from build123d import *

# Parameters (mm, degrees)
SKETCH_1_R                           = 20
EXTRUDE_1_DEPTH                      = 5
CUT_EXTRUDE_START                    = -5
SKETCH_4_R                           = 2.75
CUT_EXTRUDE_3_DEPTH                  = 15
SKETCH_7_R                           = 2.3
EXTRUDE_3_DEPTH                      = 4.5
CHAMFER_3_SIZE                       = 0.5
PATTERN_CIRCULAR_1_COUNT             = 4
CHAMFER_3_OF_PATTERN_CIRCULAR_1_SIZE = 0.5
CHAMFER_4_SIZE                       = 0.3
CHAMFER_5_SIZE                       = 1


with BuildPart() as part:
    # 草图1 → 凸台-拉伸1 (new body)
    with BuildSketch(Plane(origin=(0, 0, 0), x_dir=(1, 0, 0), z_dir=(0, 1, 0))):
        with Locations(Location((0, 0, 0), (0, 0, 270))):
            Circle(SKETCH_1_R)
    extrude(amount=EXTRUDE_1_DEPTH)

    # 草图4 → 切除-拉伸3 (cut)
    with BuildSketch(Plane(origin=(0, 5, 0), x_dir=(1, 0, 0), z_dir=(0, 1, 0)).offset(CUT_EXTRUDE_START)):
        with Locations(Location((0, 0, 0), (0, 0, 270))):
            Circle(SKETCH_4_R)
    extrude(amount=CUT_EXTRUDE_3_DEPTH, mode=Mode.SUBTRACT)

    # 草图7 → 凸台-拉伸3 (add)
    with BuildSketch(Plane(origin=(0, 5, 0), x_dir=(1, 0, 0), z_dir=(0, 1, 0))):
        with Locations(Location((6, 0, 0), (0, 0, 270))):
            Circle(SKETCH_7_R)
    extrude_3 = extrude(amount=EXTRUDE_3_DEPTH)

    # 倒角3
    chamfer_3_edges = [part.edges().sort_by_distance(p)[0] for p in [
        (6, 5, -2.3),
        (6, 9.5, -2.3),
    ]]
    chamfer(chamfer_3_edges, length=CHAMFER_3_SIZE)

    # 阵列(圆周)1: 凸台-拉伸3 ×4 about axis
    pattern_circular_1_axis = Axis((0, 0, 0), (0, 1, 0))
    for i in range(1, PATTERN_CIRCULAR_1_COUNT):
        add(extrude_3.rotate(pattern_circular_1_axis, i * 360 / PATTERN_CIRCULAR_1_COUNT))

    # 倒角3 of 阵列(圆周)1
    chamfer_3_of_pattern_circular_1_edges = [part.edges().sort_by_distance(p)[0] for p in [
        (-2.3, 5, -6),
        (-2.3, 9.5, -6),
        (-6, 5, 2.3),
        (-6, 9.5, 2.3),
        (2.3, 5, 6),
        (2.3, 9.5, 6),
    ]]
    chamfer(chamfer_3_of_pattern_circular_1_edges, length=CHAMFER_3_OF_PATTERN_CIRCULAR_1_SIZE)

    # 倒角4
    chamfer_4_edges = [part.edges().sort_by_distance(p)[0] for p in [
        (0, 5, -2.75),
        (0, 0, -2.75),
    ]]
    chamfer(chamfer_4_edges, length=CHAMFER_4_SIZE)

    # 倒角5
    chamfer_5_edges = [part.edges().sort_by_distance(p)[0] for p in [
        (0, 0, -20),
        (0, 5, -20),
    ]]
    chamfer(chamfer_5_edges, length=CHAMFER_5_SIZE)


solid = part.part
Model file for the job. Use its own axes, mm. A direction names the side the tool comes from. Give positions to 0.01 mm unless a question says otherwise; leave off trailing zeros. Loops run counter-clockwise (first coordinate to the right, second up) from the corner with the lowest first, then second, coordinate; pieces in that order, holes last. Notation, with made-up numbers: (19, -18.5) -> (33, -18.5) arc R16 cw to (33, 3.5) -> close; hole circle Ø7 at (-31.5, 40.5). An arc over 180 degrees is marked (long way). Use a Markdown table: item, result. Add a question column.
(1) Slice it at C-C on y = 3.25. List the corners of the cut face in (x, z).
(2) Wall check: line 1 along Z through (x, y) = (0, 6); line 2 along X through (y, z) = (1.7, 0); line 3 along Y through (x, z) = (16.5, 2.5). Give the ranges that are in metal, low to high.
(3) Mould opens along Z. For faces 1 (the flat face through (0, 9.5, -6)), 2 (the cylindrical face through (-19.524, 2.479, -4.336)), 3 (the cylindrical face through (0.499, 7.226, 3.755)) say: +Z half, -Z half, draft (parallel to the pull), parting line (faces both ways), or undercut.
(4) Tool access for faces 4 (the flat face through (-6, 9.5, 0)), 5 (the cylindrical face through (-0.499, 7.226, -3.755)): list every direction of +Z, -Z, +X, -X, +Y, -Y with a clear straight run to the whole face (end or side of a thin tool).
(5) Slice it at B-B on y = 7.75. List the corners of the cut face in (x, z).
(6) Drop flat-ended pins along their axis: pin 1 Ø2 at (x, z) = (12, 7.5) entering from +Y; pin 2 Ø1.5 at (x, y) = (15.5, 5.5) entering from -Z; pin 3 Ø2 at (y, z) = (6.5, 3.5) entering from -X. Give the stop position or say it passes through.
Filled sheet:
| question | item | result |
|---|---|---|
| 1 | outline | circle Ø40 at (0, 0); hole circle Ø5.5 at (0, 0) |
| 2 | line 1 | -8.3 to -3.7, 3.7 to 8.3 |
| 2 | line 2 | -20 to -2.75, 2.75 to 20 |
| 2 | line 3 | 0 to 5 |
| 3 | face 1 | draft |
| 3 | face 2 | parting line |
| 3 | face 3 | undercut |
| 4 | face 4 | +Z, -Z, +X, -X, +Y |
| 4 | face 5 | +Y |
| 5 | outline | circle Ø4.6 at (-6, 0); circle Ø4.6 at (0, -6); circle Ø4.6 at (0, 6); circle Ø4.6 at (6, 0) |
| 6 | pin 1 | y = 5 |
| 6 | pin 2 | z = -11.76 |
| 6 | pin 3 | x = -1.74 |
